Check sheet for the modelled part. Datum: model origin and axes. Units: mm. Face numbers are marked on the shaded views. A direction names the side the tool comes from. Coordinates: 2 decimals unless noted, no trailing zeros. Loops run counter-clockwise (first coordinate to the right, second up) from the corner with the lowest first, then second, coordinate; pieces in that order, holes last. Notation, with made-up numbers: (44.25, 87) - (88.25, 87) arc R15 cw to (88.25, 91) - close; hole circle Ø1 at (3.25, 70.25). An arc over 180 degrees is marked (long way). Answer as a JSON object with one key per item and string values. Group by question number.
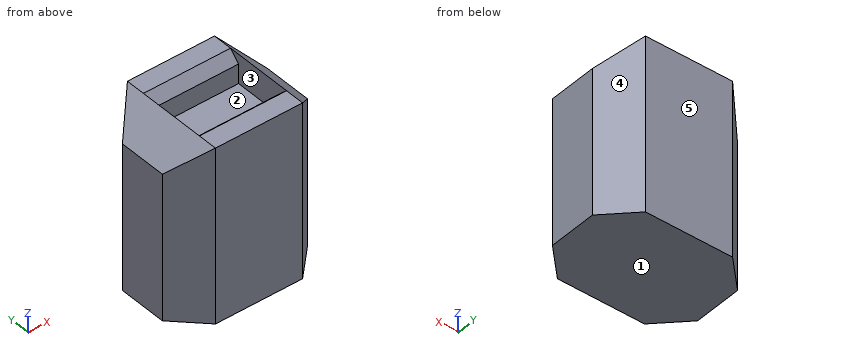
from build123d import *

# Parameters (mm, degrees)
F0_W     = 45
F0_H     = 25
F1_DEPTH = 75
F2_DEPTH = 90
F3_SIZE  = 14.99999
F4_SIZE  = 5


# Not quite as in the source:
# - a fillet or chamfer is up to 0.001 mm smaller than in the source, because OpenCascade refuses the exact size


with BuildPart() as f1:
    # F0 (on Top) → F1 (new body)
    with BuildSketch(Plane.XY):
        Rectangle(F0_W, F0_H)
    extrude(amount=F1_DEPTH)

    # F0 (on Top) → F2 (join)
    with BuildSketch(Plane.XY):
        Polygon((37.5, 27.5), (-37.5, 27.5), (-37.5, -27.5), (-22.5, -27.5), (22.5, -27.5), (37.5, -27.5), align=None)
        Rectangle(F0_W, F0_H, mode=Mode.SUBTRACT)
    extrude(amount=F2_DEPTH)

    # F3 (size 15 in the source; OpenCascade refuses exactly that, so slightly less here)
    f3_edges = [f1.edges().sort_by_distance(p)[0] for p in [
        (-37.5, 0, 90),
        (37.5, 0, 90),
        (37.5, 27.5, 45),
        (37.5, -27.5, 45),
        (-37.5, -27.5, 45),
        (-37.5, 27.5, 45),
    ]]
    chamfer(f3_edges, length=F3_SIZE)

    # F4
    f4_edges = [f1.edges().sort_by_distance(p)[0] for p in [
        (0, 12.5, 90),
        (0, -12.5, 90),
    ]]
    chamfer(f4_edges, length=F4_SIZE)


solid = f1.part
1. Sectioned sample at C-C on z = 70.5. Record the cut outline in (x, y).
2. Gauge pin test, flat ends, axial feed: pin 1 (1.5 mm diameter, centred on y = 15.5, z = 79, fed in from -X); pin 2 (16.5 mm diameter, centred on y = 1, z = 85.5, fed in from +X). Record the tip position at first contact, or that the pin passes through.
3. Access from +Z, -Z, +X, -X, +Y, -Y to the whole of each face (thin tool, end or side, straight path). Record for the marked faces 1 and 2.
4. Sectioned sample at D-D on x = -9. Record the cut outline in (y, z).
5. Sectioned sample at B-B on z = 79.5. Record the cut outline in (x, y).
6. Material ranges on line 1 (Y direction, x = -9.5, z = 81); line 2 (Z direction, x = -9, y = 4.5); line 3 (X direction, y = -1, z = 82), recorded low to high.
7. Release check for a two-part mould opening along X. For the marked faces 3, 4 and 5 record: released by +X, released by -X, zero draft, split by the parting line, or undercut.
Answers follow:
{
 "1": {"outline": "(-37.5, -12.5) - (-22.5, -27.5) - (22.5, -27.5) - (37.5, -12.5) - (37.5, 12.5) - (22.5, 27.5) - (-22.5, 27.5) - (-37.5, 12.5) - close"},
 "2": {"pin 1": "stops at x = -34.25", "pin 2": "stops at x = 35.25"},
 "3": {"face 1": "-Z, +X, -X, +Y, -Y", "face 2": "+Z"},
 "4": {"outline": "(-27.5, 0) - (27.5, 0) - (27.5, 90) - (17.5, 90) - (12.5, 85) - (12.5, 75) - (-12.5, 75) - (-12.5, 85) - (-17.5, 90) - (-27.5, 90) - close"},
 "5": {"outline": "(-33, -17) - (-22.5, -27.5) - (22.5, -27.5) - (33, -17) - (33, 17) - (22.5, 27.5) - (-22.5, 27.5) - (-33, 17) - close; hole (-22.5, -12.5) - (22.5, -12.5) - (22.5, 12.5) - (-22.5, 12.5) - close"},
 "6": {"line 1": "y = -27.5 to -12.5, 12.5 to 27.5", "line 2": "z = 0 to 75", "line 3": "x = -30.5 to -22.5, 22.5 to 30.5"},
 "7": {"face 3": "undercut", "face 4": "released by +X", "face 5": "zero draft"}
}
